from build123d import *

# Parameters (mm, degrees)
SKETCH1_W           = 15
SKETCH1_H           = 8
SKETCH1_R           = 1.5
BOSS_EXTRUDE1_DEPTH = 3
SKETCH2_W           = 12.5
SKETCH2_H           = 8
SKETCH2_R           = 1.5
BOSS_EXTRUDE2_DEPTH = 3
CHAMFER1_SIZE       = 2


with BuildPart() as part:
    # Sketch1 → Boss-Extrude1 (new body)
    with BuildSketch(Plane(origin=(0, 0, 0), x_dir=(0, 0, -1), z_dir=(1, 0, 0))):
        with Locations((7.5, -4)):
            Rectangle(SKETCH1_W, SKETCH1_H)
        with Locations((4, -4)):
            Circle(SKETCH1_R, mode=Mode.SUBTRACT)
    extrude(amount=BOSS_EXTRUDE1_DEPTH)

    # Sketch2 → Boss-Extrude2 (add)
    with BuildSketch(Plane(origin=(0, 0, -15), x_dir=(-1, 0, 0), z_dir=(0, 0, -1))):
        with Locations((-6.25, -4)):
            Rectangle(SKETCH2_W, SKETCH2_H)
        with Locations(Location((-8.5, -4, 0), (0, 0, 90))):
            Circle(SKETCH2_R, mode=Mode.SUBTRACT)
    extrude(amount=-BOSS_EXTRUDE2_DEPTH)

    # Chamfer1
    chamfer1_edges = [part.edges().sort_by_distance(p)[0] for p in [
        (3, -4, -12),
    ]]
    chamfer(chamfer1_edges, length=CHAMFER1_SIZE)


solid = part.part
The listing builds one solid part. Answer for the finished solid, in the listing's coordinates (mm). A direction names the side the tool comes from. Coordinates: 2 decimals unless noted, no trailing zeros. Write each loop counter-clockwise with the first axis right and the second up, starting at its lowest first coordinate (ties: lowest second). Pieces come first, ordered by that corner, then holes. Notation, with made-up numbers: (30.5, -20) - (67.5, -20) arc R21 ccw to (67.5, 13) - close; hole circle Ø1 at (-21, -30.5). An arc over 180 degrees is marked (long way). Put each result on its own line as item: value.
1. The part is cut by section A-A on y = -4. Give the vertices of the cut face in (x, z).
Answer sheet:
outline: (0, -15) - (7, -15) - (7, -12) - (5, -12) - (3, -10) - (3, -5.5) - (0, -5.5) - close; (0, -2.5) - (3, -2.5) - (3, 0) - (0, 0) - close; (10, -15) - (12.5, -15) - (12.5, -12) - (10, -12) - close
2. The part is cut by section D-D on y = -5.75. Give the vertices of the cut face in (x, z).
Answer sheet:
outline: (0, -15) - (12.5, -15) - (12.5, -12) - (5, -12) - (3, -10) - (3, 0) - (0, 0) - close
3. Find the intervals of material crossed by line 1 along X through (y, z) = (-4, -13.45); line 2 along Y through (x, z) = (1.95, -4); line 3 along Z through (x, y) = (8, -1.5), in increasing order. Write a range as from..to.
Answer sheet:
line 1: x = 0..7, 10..12.5
line 2: y = -8..-5.5, -2.5..0
line 3: z = -15..-12
4. A tool of negligible diameter and unlimited length cuts with its end or side. For faces 4 (the face through (3, -4, -6)), 5 (the face through (12.5, -4, -14)), from which of +Z, -Z, +X, -X, +Y, -Y can it reach the whole face along a straight path? Write none if from no direction.
Answer sheet:
face 4: +Z, +X, +Y, -Y
face 5: +Z, -Z, +X, +Y, -Y
5. The part is cut by section C-C on z = -4. Give the vertices of the cut face in (x, y), plus the area to 3 significant figures.
Answer sheet:
outline: (0, -8) - (3, -8) - (3, -5.5) - (0, -5.5) - close; (0, -2.5) - (3, -2.5) - (3, 0) - (0, 0) - close
area: 15.0 mm^2
6. Flat-ended cylindrical pins translate along their axes: pin 1 Ø1 at (y, z) = (-1.5, -5) entering from +X; pin 2 Ø4 at (x, y) = (8.5, -4) entering from +Z; pin 3 Ø2 at (x, y) = (5, -5) entering from +Z. Find the tip coordinate at first contact, or state that the pin passes through.
Answer sheet:
pin 1: stops at x = 3
pin 2: stops at z = -12
pin 3: stops at z = -11
7. The part is cut by section B-B on x = 8.5. Give the vertices of the cut face in (y, z).
Answer sheet:
outline: (-8, -15) - (-5.5, -15) - (-5.5, -12) - (-8, -12) - close; (-2.5, -15) - (0, -15) - (0, -12) - (-2.5, -12) - close
8. Determine the mould class of faces 1 (the face through (1, -4, 0)), 2 (the face through (7.17, -3.31, -13.52)), 3 (the face through (0, -4, -7)) for opening direction X: pulls with the +X half, pulls with the -X half, needs draft (parallel to the pull), parting line crosses it, or undercut.
Answer sheet:
face 1: needs draft
face 2: undercut
face 3: pulls with the -X half
